```python
from build123d import *

# Parameters (mm, degrees)
BOSS_EXTRU_1_DEPTH        = 13
COQUE1_T                  = -5
COQUE1_THICKNESS_2_FACE_W = 65
COQUE1_THICKNESS_2_FACE_H = 65
COQUE1_THICKNESS_2_DEPTH  = 2
ENL_V_MAT_EXTRU_1_REACH   = 88.587
ESQUISSE2_R               = 2.5
ENL_V_MAT_EXTRU_2_REACH   = 95.396
ESQUISSE3_R               = 2.5
ESQUISSE4_W               = 18
ESQUISSE4_H               = 18
ESQUISSE4_W_2             = 15
ESQUISSE4_H_2             = 15
BOSS_EXTRU_2_DEPTH        = 10
ESQUISSE5_R               = 11.5
ESQUISSE5_R_2             = 14.5
ENL_V_MAT_EXTRU_3_DEPTH   = 13
ESQUISSE6_R               = 5
ENL_V_MAT_EXTRU_4_DEPTH   = 3


with BuildPart() as part:
    # Esquisse1 → Boss.-Extru.1 (new body)
    with BuildSketch(Plane.XY):
        Polygon((44.118436308, 33.728448276), (54.118436308, 33.728448276), (54.118436308, 23.728448276), (54.118436308, -41.271551724), (-20.881563692, -41.271551724), (-20.881563692, 33.728448276), align=None)
    extrude(amount=BOSS_EXTRU_1_DEPTH)

    # Coque1
    coque1_openings = [part.faces().sort_by_distance(p)[0] for p in [
        (16.618436308, -3.771551724, 13),
    ]]
    offset(amount=COQUE1_T, openings=coque1_openings, kind=Kind.INTERSECTION)

    # Coque1 thickness 2 face (on inner face of the shell) → Coque1 thickness 2 (cut)
    with BuildSketch(Plane(origin=(16.618436308, -3.771551724, 5), x_dir=(-1, 0, 0), z_dir=(0, 0, -1))):
        Rectangle(COQUE1_THICKNESS_2_FACE_W, COQUE1_THICKNESS_2_FACE_H)
    extrude(amount=COQUE1_THICKNESS_2_DEPTH, mode=Mode.SUBTRACT)

    # Enlèv. mat.-Extru.1: up to this face of the body (flat: up to its plane)
    enl_v_mat_extru_1_end = Plane(part.part.faces().sort_by_distance((54.118436308, -3.771551724, 6.5))[0])
    # Esquisse2 → Enlèv. mat.-Extru.1 (cut, up to the picked face)
    with BuildSketch(Plane.ZY.offset(20.881563692), mode=Mode.PRIVATE) as enl_v_mat_extru_1_sk1:
        with Locations(Location((8, -16.271551724, 0), (0, 0, 270))):
            Circle(ESQUISSE2_R)
    enl_v_mat_extru_1_tool1 = split(extrude(enl_v_mat_extru_1_sk1.sketch, amount=-ENL_V_MAT_EXTRU_1_REACH, mode=Mode.PRIVATE), bisect_by=enl_v_mat_extru_1_end, keep=Keep.BOTH, mode=Mode.PRIVATE)
    # Esquisse2 → Enlèv. mat.-Extru.1 (cut, up to the picked face)
    with BuildSketch(Plane.ZY.offset(20.881563692), mode=Mode.PRIVATE) as enl_v_mat_extru_1_sk2:
        with Locations(Location((8, 8.728448276, 0), (0, 0, 270))):
            Circle(ESQUISSE2_R)
    enl_v_mat_extru_1_tool2 = split(extrude(enl_v_mat_extru_1_sk2.sketch, amount=-ENL_V_MAT_EXTRU_1_REACH, mode=Mode.PRIVATE), bisect_by=enl_v_mat_extru_1_end, keep=Keep.BOTH, mode=Mode.PRIVATE)
    add(enl_v_mat_extru_1_tool1.solids().sort_by(Axis((-20.881564, -16.271552, 8), (1, 0, 0)))[0], mode=Mode.SUBTRACT)
    add(enl_v_mat_extru_1_tool2.solids().sort_by(Axis((-20.881564, 8.728448, 8), (1, 0, 0)))[0], mode=Mode.SUBTRACT)

    # Enlèv. mat.-Extru.2: up to this face of the body (flat: up to its plane)
    enl_v_mat_extru_2_end = Plane(part.part.faces().sort_by_distance((16.618436308, 33.728448276, 6.5))[0])
    # Esquisse3 → Enlèv. mat.-Extru.2 (cut, up to the picked face)
    with BuildSketch(Plane.XZ.offset(41.271551724), mode=Mode.PRIVATE) as enl_v_mat_extru_2_sk1:
        with Locations(Location((4.118436308, 8, 0), (0, 0, 270))):
            Circle(ESQUISSE3_R)
    enl_v_mat_extru_2_tool1 = split(extrude(enl_v_mat_extru_2_sk1.sketch, amount=-ENL_V_MAT_EXTRU_2_REACH, mode=Mode.PRIVATE), bisect_by=enl_v_mat_extru_2_end, keep=Keep.BOTH, mode=Mode.PRIVATE)
    # Esquisse3 → Enlèv. mat.-Extru.2 (cut, up to the picked face)
    with BuildSketch(Plane.XZ.offset(41.271551724), mode=Mode.PRIVATE) as enl_v_mat_extru_2_sk2:
        with Locations(Location((29.118436308, 8, 0), (0, 0, 270))):
            Circle(ESQUISSE3_R)
    enl_v_mat_extru_2_tool2 = split(extrude(enl_v_mat_extru_2_sk2.sketch, amount=-ENL_V_MAT_EXTRU_2_REACH, mode=Mode.PRIVATE), bisect_by=enl_v_mat_extru_2_end, keep=Keep.BOTH, mode=Mode.PRIVATE)
    add(enl_v_mat_extru_2_tool1.solids().sort_by(Axis((4.118436, -41.271552, 8), (0, 1, 0)))[0], mode=Mode.SUBTRACT)
    add(enl_v_mat_extru_2_tool2.solids().sort_by(Axis((29.118436, -41.271552, 8), (0, 1, 0)))[0], mode=Mode.SUBTRACT)

    # Esquisse4 → Boss.-Extru.2 (add)
    with BuildSketch(Plane.XY.offset(3)):
        Polygon((-5.881563692, 28.728448276), (-15.881563692, 18.728448276), (-15.881563692, 28.728448276), align=None)
        Polygon((49.118436308, 28.728448276), (49.118436308, 18.728448276), (39.118436308, 28.728448276), align=None)
        with Locations((45.118436308, -32.271551724)):
            Rectangle(ESQUISSE4_W, ESQUISSE4_H)
        with Locations((-13.381563692, -33.771551724)):
            Rectangle(ESQUISSE4_W_2, ESQUISSE4_H_2)
    extrude(amount=BOSS_EXTRU_2_DEPTH)

    # Esquisse5 → Enlèv. mat.-Extru.3 (cut)
    with BuildSketch(Plane.XY.offset(13)):
        with Locations((-20.881563692, -41.271551724)):
            Circle(ESQUISSE5_R)
        with Locations((54.118436308, -41.271551724)):
            Circle(ESQUISSE5_R_2)
    extrude(amount=-ENL_V_MAT_EXTRU_3_DEPTH, mode=Mode.SUBTRACT)

    # Esquisse6 → Enlèv. mat.-Extru.4 (cut)
    with BuildSketch(Plane.XY.offset(3)):
        with Locations((-0.881563692, 13.728448276)):
            Circle(ESQUISSE6_R)
    extrude(amount=-ENL_V_MAT_EXTRU_4_DEPTH, mode=Mode.SUBTRACT)


solid = part.part
```
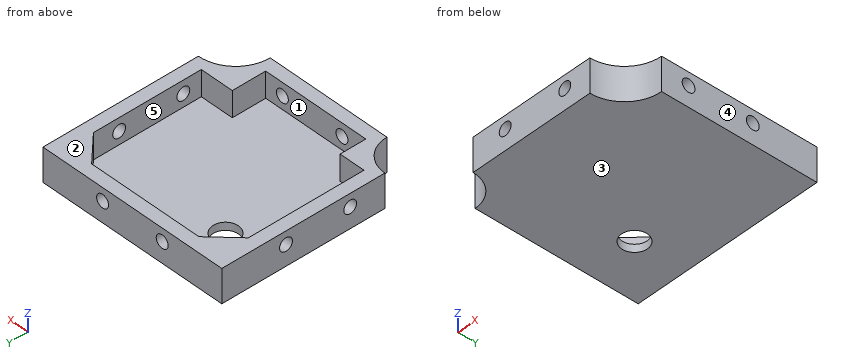
Input: part model. Units: mm. Frame: model coordinates. Face numbers are marked on the shaded views. A direction names the side the tool comes from. Give positions to 0.01 mm unless a question says otherwise; leave off trailing zeros. Order: outer loops, then holes, each group sorted by start corner. A loop starts at its lowest first (then second) coordinate and runs counter-clockwise, first axis right, second up.
1. Cut plane B-B (y = 2). Return loops of the section in (x, z), and give its area (3 significant figures).
Computed:
outline: (-20.88, 0) - (54.12, 0) - (54.12, 13) - (49.12, 13) - (49.12, 3) - (-15.88, 3) - (-15.88, 13) - (-20.88, 13) - close
area: 325 mm2
2. Cut plane A-A (z = 12). Return loops of the section in (x, y).
Computed:
outline: (-20.88, -29.77) arc R11.5 cw to (-9.38, -41.27) - (39.62, -41.27) arc R14.5 cw to (54.12, -26.77) - (54.12, 33.73) - (-20.88, 33.73) - close; hole (-15.88, -26.27) - (-5.88, -26.27) - (-5.88, -36.27) - (36.12, -36.27) - (36.12, -23.27) - (49.12, -23.27) - (49.12, 18.73) - (39.12, 28.73) - (-5.88, 28.73) - (-15.88, 18.73) - close
3. Line query: probe 1 along X at (y, z) = (31.6, 8); probe 2 along X at (y, z) = (-4, 8.5); probe 3 along Y at (x, z) = (1, 12.25). Output: solid intervals per line, ascending.
Computed:
probe 1: x = -20.88 to 1.62, 6.62 to 26.62, 31.62 to 54.12
probe 2: x = -20.88 to -15.88, 49.12 to 54.12
probe 3: y = -41.27 to -36.27, 28.73 to 33.73
4. Cut plane C-C (x = 10.5). Return loops of the section in (y, z), and give its area (3 significant figures).
Computed:
outline: (-41.27, 0) - (33.73, 0) - (33.73, 13) - (28.73, 13) - (28.73, 3) - (-36.27, 3) - (-36.27, 13) - (-41.27, 13) - close
area: 325 mm2
5. Pin query (flat end, axial travel): pin 1 Ø10 at (x, y) = (14, -30) entering from +Z; pin 2 Ø10 at (x, y) = (5, 25) entering from +Z; pin 3 Ø3 at (x, z) = (29.12, 8) entering from +Y; pin 4 Ø5 at (y, z) = (-31, 7.5) entering from +X. Return the tip coordinate at first contact, or that it passes through.
Computed:
pin 1: stops at z = 3
pin 2: stops at z = 13
pin 3: passes through
pin 4: stops at x = 47.25
6. Draft query along X for the marked faces 3, 4 and 5. Return one class per face: released by +X, released by -X, zero draft, split by the parting line, or undercut.
Computed:
face 3: zero draft
face 4: released by +X
face 5: undercut
7. Set-up query: the marked faces 1 and 2. Return all of +Z, -Z, +X, -X, +Y, -Y with unobstructed straight access to the full face (end or side cutting, diameter ignored); none if empty.
Computed:
face 1: +Z
face 2: +Z, +X, -X, +Y, -Y
8. Cut plane D-D (z = 8). State how many separate pieces and enclosed holes the cut face has, and give its area (3 significant figures).
Computed:
separate pieces: 8
enclosed holes: 0
area: 1,300 mm2
